from build123d import *

# Parameters (mm, degrees)
DODANIE_WYCI_GNI_CIE1_DEPTH = 5
SZKIC2_W                    = 100
SZKIC2_H                    = 35
DODANIE_WYCI_GNI_CIE2_DEPTH = 5
SZKIC3_R                    = 6
WYTNIJ_WYCI_GNI_CIE1_DEPTH  = 99.234413522
SZKIC4_W                    = 100
SZKIC4_H                    = 40
DODANIE_WYCI_GNI_CIE3_DEPTH = 5


with BuildPart() as part:
    # Szkic1 → Dodanie-wyci_gni_cie1 (new body)
    with BuildSketch(Plane.XY):
        with BuildLine():
            Line((-65, -20), (65, -20))
            Line((65, -20), (65, 20))
            Line((65, 20), (-65, 20))
            ThreePointArc((-65, 20), (-85, 0), (-65, -20))
        make_face()
    extrude(amount=DODANIE_WYCI_GNI_CIE1_DEPTH)


with BuildPart() as body_2:
    # Lustro2: mirrored copy
    add(part.part.mirror(Plane.XY.offset(22.5)))


with BuildPart() as part_1:
    add(part.part)

    add(body_2.part)  # Dodanie-wyci_gni_cie2 merges body 2
    # Szkic2 → Dodanie-wyci_gni_cie2 (add)
    with BuildSketch(Plane(origin=(0, 20, 0), x_dir=(1, 0, 0), z_dir=(0, 1, 0))):
        with Locations((15, -22.5)):
            Rectangle(SZKIC2_W, SZKIC2_H)
    extrude(amount=-DODANIE_WYCI_GNI_CIE2_DEPTH)

    # Szkic3 → Wytnij-wyci_gni_cie1 (cut, through all)
    with BuildSketch(Plane(origin=(0, 0, 0), x_dir=(-1, 0, 0), z_dir=(0, 0, -1))):
        with Locations((65, 0)):
            Circle(SZKIC3_R)
    extrude(amount=-WYTNIJ_WYCI_GNI_CIE1_DEPTH, mode=Mode.SUBTRACT)

    # Szkic4 → Dodanie-wyci_gni_cie3 (add)
    with BuildSketch(Plane.XZ.offset(20)):
        with Locations((15, 20)):
            Rectangle(SZKIC4_W, SZKIC4_H)
    extrude(amount=-DODANIE_WYCI_GNI_CIE3_DEPTH)


solid = part_1.part
Could you check a few things on this model? Use its own coordinates, in mm. A direction names the side the tool comes from. Give positions to 0.01 mm unless a question says otherwise; leave off trailing zeros. Order: outer loops, then holes, each group sorted by start corner. A loop starts at its lowest first (then second) coordinate and runs counter-clockwise, first axis right, second up.
1. Will these pins go through, and if not, where does the flat tip stop? P1, Ø5, axis at y = 11, z = 15.5, coming from the +X side; P2, Ø1.5, axis at y = 17, z = 26, coming from the -X side; P3, Ø6, axis at x = -67, z = 39.5, coming from the -Y side.
2. I need wall thicknesses on L1, parallel to Z at x = 56.5, y = -10.5; L2, parallel to Y at x = -65, z = 1; L3, parallel to Y at x = 32, z = 8.5. Which ranges of each line are inside material? Lowest first, please.
3. Suppose I cut it at B-B (x = -57). List the corners of the cut face in (y, z) for me, plus the area to 3 significant figures.
4. For faces 5 (the flat face through (14, -15, 23)), 6 (the flat face through (-35, -18, 22)), 7 (the flat face through (14, 20, 22)), which set-ups out of +Z, -Z, +X, -X, +Y, -Y let a thin tool reach every point of the face, with its end or its side?
5. Suppose I cut it at D-D (x = 14.5). List the corners of the cut face in (y, z) for me.
6. We'd pull the mould along Y, two halves only. Please class faces 1 (the cylindrical face through (-85, 0, 2)), 2 (the flat face through (-11, 0, 40)), 3 (the flat face through (-11, 0, 45)), 4 (the flat face through (14, 15, 22)): pulls with the +Y half, pulls with the -Y half, needs draft (parallel to the pull), parting line crosses it, or undercut.
7. Suppose I cut it at C-C (z = 21). List the corners of the cut face in (x, y) for me.
8. Suppose I cut it at A-A (y = 0). List the corners of the cut face in (x, z) for me, plus the area to 3 significant figures.
Solved:
1. P1: passes through
1. P2: stops at x = -35
1. P3: stops at y = -20
2. L1: z = 0 to 5, 40 to 45
2. L2: y = -20 to -6, 6 to 20
2. L3: y = -20 to -15, 15 to 20
3. outline: (-20, 0) - (20, 0) - (20, 5) - (-20, 5) - close; (-20, 40) - (20, 40) - (20, 45) - (-20, 45) - close
3. area: 400 mm2
4. face 5: +X, -X
4. face 6: -X, +Y, -Y
4. face 7: +Z, -Z, +X, -X, +Y
5. outline: (-20, 0) - (20, 0) - (20, 45) - (-20, 45) - close; hole (-15, 5) - (15, 5) - (15, 40) - (-15, 40) - close
6. face 1: parting line crosses it
6. face 2: undercut
6. face 3: needs draft
6. face 4: undercut
7. outline: (-35, -20) - (65, -20) - (65, -15) - (-35, -15) - close; (-35, 15) - (65, 15) - (65, 20) - (-35, 20) - close
8. outline: (-85, 0) - (-71, 0) - (-71, 5) - (-85, 5) - close; (-85, 40) - (-71, 40) - (-71, 45) - (-85, 45) - close; (-59, 0) - (65, 0) - (65, 5) - (-59, 5) - close; (-59, 40) - (65, 40) - (65, 45) - (-59, 45) - close
8. area: 1,380 mm2
